Verification items for the finished model (mm, model axes). Coordinates: 2 decimals unless noted, no trailing zeros. Order: outer loops, then holes, each group sorted by start corner. A loop starts at its lowest first (then second) coordinate and runs counter-clockwise, first axis right, second up. Notation, with made-up numbers: M 53.25,35 L 70.25,35 A26 ccw 70.25,59 Z; hole C 85.5,70 d2. An arc over 180 degrees is marked long. Answer as a JSON object with one key per item and string values. Group by question number.
(1) Gauge pin test, flat end, axial feed: pin 1 Ø1.5 at (y, z) = (5, 39.5) entering from +X. Record the tip position at first contact, or that the pin passes through.
(2) Cross-section at A-A (z = 15). Enter the section's corners in (x, y), plus the area to 3 significant figures.
(3) Material ranges on line 1 (X direction, y = 3.95, z = 102.5); line 2 (X direction, y = 2.8, z = 80); line 3 (Y direction, x = -1.5, z = 133.5), recorded low to high.
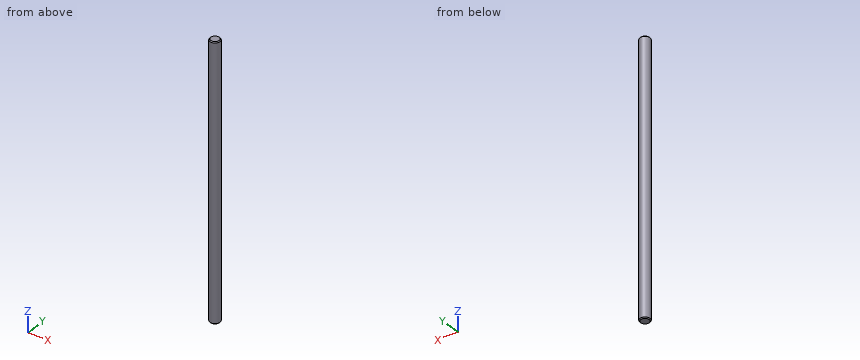
from build123d import *

# Parameters (mm, degrees)
SKETCH1_R           = 3
BOSS_EXTRUDE1_DEPTH = 160
CHAMFER1_SIZE       = 0.5
CHAMFER2_SIZE       = 0.5


with BuildPart() as part:
    # Sketch1 → Boss-Extrude1 (new body)
    with BuildSketch(Plane.XY):
        with Locations((0, 3.620771249)):
            Circle(SKETCH1_R)
    extrude(amount=BOSS_EXTRUDE1_DEPTH)

    # Chamfer1
    chamfer1_edges = [part.edges().sort_by_distance(p)[0] for p in [
        (-3, 3.620771249, 160),
    ]]
    chamfer(chamfer1_edges, length=CHAMFER1_SIZE)

    # Chamfer2
    chamfer2_edges = [part.edges().sort_by_distance(p)[0] for p in [
        (-3, 3.620771249, 0),
    ]]
    chamfer(chamfer2_edges, length=CHAMFER2_SIZE)


solid = part.part
Taken from the geometry:
{
 "1": {"pin 1": "stops at x = 2.93"},
 "2": {"outline": "C 0,3.62 d6", "area": "28.3 mm²"},
 "3": {"line 1": "x = -2.98 to 2.98", "line 2": "x = -2.89 to 2.89", "line 3": "y = 1.02 to 6.22"}
}
